```python
from build123d import *

# Parameters (mm, degrees)
SKETCH_1_W                   = 40
SKETCH_1_H                   = 40
SKETCH_1_R                   = 5.2
SKETCH_1_R_2                 = 1.6
EXTRUDE_1_DEPTH              = 5
HOLE_WIZARD_1_D              = 3
CHAMFER_1_SIZE               = 2
HOLE_WIZARD_M3_2_D           = 3.4
HOLE_WIZARD_M3_2_CSINK_D     = 6.6
HOLE_WIZARD_M3_2_CSINK_ANGLE = 90
SKETCH_7_R                   = 2.5
EXTRUDE_2_DEPTH              = 5
SKETCH_10_W                  = 9
SKETCH_10_H                  = 7
SKETCH_10_R                  = 1.5
EXTRUDE_4_DEPTH              = 4
EXTRUDE_6_DEPTH              = 3


with BuildPart() as part:
    # 草图1 → 凸台-拉伸1 (new body)
    with BuildSketch(Plane.XY):
        Rectangle(SKETCH_1_W, SKETCH_1_H)
        Circle(SKETCH_1_R, mode=Mode.SUBTRACT)
        with Locations((5.656854249, 5.656854249)):
            Circle(SKETCH_1_R_2, mode=Mode.SUBTRACT)
        with Locations((5.656854249, -5.656854249)):
            Circle(SKETCH_1_R_2, mode=Mode.SUBTRACT)
        with Locations((-5.656854249, -5.656854249)):
            Circle(SKETCH_1_R_2, mode=Mode.SUBTRACT)
        with Locations((-5.656854249, 5.656854249)):
            Circle(SKETCH_1_R_2, mode=Mode.SUBTRACT)
    extrude(amount=EXTRUDE_1_DEPTH)

    # 孔1 (through all)
    with Locations(Plane(origin=(16.25, -4, 5), x_dir=(1, 0, 0), z_dir=(0, 0, 1))):
        with Locations((0, 0), (-32.5, 0)):
            Hole(HOLE_WIZARD_1_D / 2)

    # 倒角1
    chamfer_1_edges = [part.edges().sort_by_distance(p)[0] for p in [
        (20, 20, 2.5),
    ]]
    chamfer(chamfer_1_edges, length=CHAMFER_1_SIZE)

    # M3 十字槽沉头木螺钉的锥形沉头孔2 (through all)
    with Locations(Plane.XY.offset(5)):
        with Locations((-5.656854249, 5.656854249), (5.656854249, 5.656854249), (5.656854249, -5.656854249), (-5.656854249, -5.656854249)):
            CounterSinkHole(HOLE_WIZARD_M3_2_D / 2, HOLE_WIZARD_M3_2_CSINK_D / 2, counter_sink_angle=HOLE_WIZARD_M3_2_CSINK_ANGLE)

    # 草图7 → 凸台-拉伸2 (add)
    with BuildSketch(Plane(origin=(0, 0, 0), x_dir=(-1, 0, 0), z_dir=(0, 0, -1))):
        Polygon((-11.507772726, 20), (-6.507772726, 20), (6.507772726, 20), (11.507772726, 20), (6.507772726, 32), (-6.507772726, 32), align=None)
        with Locations((0, 26)):
            Circle(SKETCH_7_R, mode=Mode.SUBTRACT)
    extrude(amount=-EXTRUDE_2_DEPTH)

    # 草图10 → 凸台-拉伸4 (add)
    with BuildSketch(Plane.XZ.offset(20)):
        with Locations((15.5, -3.5)):
            Rectangle(SKETCH_10_W, SKETCH_10_H)
        with Locations(Location((17, -4, 0), (0, 0, 270))):
            Circle(SKETCH_10_R, mode=Mode.SUBTRACT)
    extrude_4 = extrude(amount=-EXTRUDE_4_DEPTH)

    # 草图12 → 凸台-拉伸6 (add)
    with BuildSketch(Plane.ZY.offset(-11)):
        Polygon((-7, -16), (0, -9), (0, -16), align=None)
    extrude_6 = extrude(amount=-EXTRUDE_6_DEPTH)

    # 镜向2: 凸台-拉伸4, 凸台-拉伸6 across plane
    add(extrude_4.mirror(Plane(origin=(0, 0, 0), x_dir=(0, 0, 1), z_dir=(1, 0, 0))))
    add(extrude_6.mirror(Plane(origin=(0, 0, 0), x_dir=(0, 0, 1), z_dir=(1, 0, 0))))


solid = part.part
```
Check sheet for the modelled part. Datum: model origin and axes. Units: mm. A direction names the side the tool comes from. Coordinates: 2 decimals unless noted, no trailing zeros. Write each loop counter-clockwise with the first axis right and the second up, starting at its lowest first coordinate (ties: lowest second). Pieces come first, ordered by that corner, then holes. Notation, with made-up numbers: M 79,49.25 L 124,49.25 A14 ccw 124,65.25 Z; hole C -22.5,5.25 d6. An arc over 180 degrees is marked long. Write item = value, one per line. Start each with the question number.
1. Sectioned sample at C-C (x = 17). Record the cut outline in (y, z).
2. Sectioned sample at A-A (z = -4). Record the cut outline in (x, y).
3. Thickness scan on probe 1 along Y at (x, z) = (0, 2.5); probe 2 along Y at (x, z) = (6, 2.5); probe 3 along Z at (x, y) = (-17, -18.05). Record the ranges inside material, lowest first.
4. Sectioned sample at D-D (x = 12.5). Record the cut outline in (y, z), then the cut area to 4 significant figures.
5. Go/stop test with flat-tipped pins: pin 1 (2.5 mm diameter, centred on x = -5.66, y = -5.66, fed in from -Z); pin 2 (20 mm diameter, centred on x = -6.5, y = 19, fed in from -Z); pin 3 (5.5 mm diameter, centred on x = 5.66, y = 5.66, fed in from +Z); pin 4 (1.5 mm diameter, centred on x = -15.5, z = -2, fed in from +Y). Record where each tip stops, or that it passes through.
6. Sectioned sample at B-B (y = 0). Record the cut outline in (x, z).
7. Mould release check, pull along X, two halves, no side actions. Record for faces 4 (the conical face through (-6.71, 7.31, 3.66)), 5 (the flat face through (-20, 0, 2)), 6 (the cylindrical face through (4.96, 1.56, 2.47)), 7 (the flat face through (8.973, 26.084, 2.465)): pulls with the +X half, pulls with the -X half, needs draft (parallel to the pull), parting line crosses it, or undercut.
8. Tool access check on faces 1 (the flat face through (-11, -16, -3)), 2 (the flat face through (-16, 20, 2)), 3 (the flat face through (-17, -16, -2)). Record the directions out of +Z, -Z, +X, -X, +Y, -Y that give a thin tool (end or side, any length) a straight path to the whole face; none if there is none.
The answers:
q1.outline = M -20,-7 L -16,-7 L -16,-5.5 L -20,-5.5 Z; M -20,-2.5 L -16,-2.5 L -16,0 L -5.3,0 L -5.3,5 L -20,5 Z; M -2.7,0 L 20,0 L 20,5 L -2.7,5 Z
q2.outline = M -20,-20 L -18.5,-20 L -18.5,-16 L -20,-16 Z; M -15.5,-20 L -11,-20 L -11,-13 L -14,-13 L -14,-16 L -15.5,-16 Z; M 11,-20 L 15.5,-20 L 15.5,-16 L 14,-16 L 14,-13 L 11,-13 Z; M 18.5,-20 L 20,-20 L 20,-16 L 18.5,-16 Z
q3.probe_1 = -20 to -5.2, 5.2 to 23.5, 28.5 to 32
q3.probe_2 = -20 to -7.32, -3.99 to 3.99, 7.32 to 32
q3.probe_3 = -7 to -5.5, -2.5 to 5
q4.outline = M -20,-7 L -16,-7 L -9,0 L 20,0 L 20,5 L -20,5 Z
q4.area = 252.5 mm²
q5.pin_1 = through
q5.pin_2 = 0
q5.pin_3 = 4.45
q5.pin_4 = -16
q6.outline = M -20,0 L -5.2,0 L -5.2,5 L -20,5 Z; M 5.2,0 L 20,0 L 20,5 L 5.2,5 Z
q7.face_4 = undercut
q7.face_5 = pulls with the -X half
q7.face_6 = undercut
q7.face_7 = pulls with the +X half
q8.face_1 = -Z, +Y, -Y
q8.face_2 = +Z, -Z, -X, +Y
q8.face_3 = -Z, -X, +Y
